Source: CAD feature listing. Evaluate the final solid. Frame: model axes, mm. Face numbers are marked on the shaded views. A direction names the side the tool comes from. Coordinates: 2 decimals unless noted, no trailing zeros. Order: outer loops, then holes, each group sorted by start corner. A loop starts at its lowest first (then second) coordinate and runs counter-clockwise, first axis right, second up. Notation, with made-up numbers: (32.5, -8.5) -> (61.5, -8.5) arc R26 cw to (61.5, 24.5) -> close; hole circle Ø5 at (13, 14). An arc over 180 degrees is marked (long way). Write each question's results on one line, items separated by ' | '. Start each with the question number.
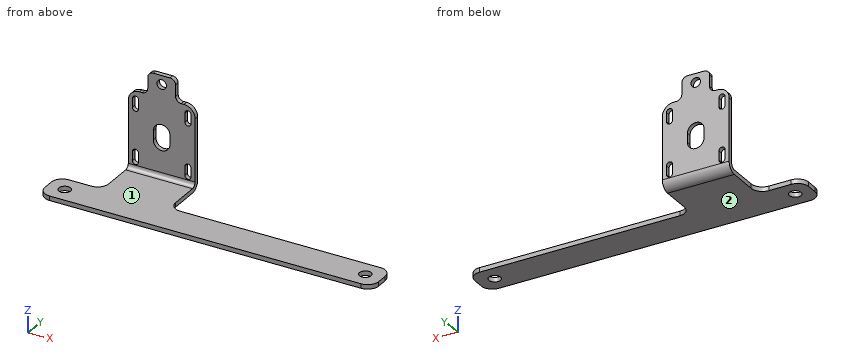
from build123d import *

# Parameters (mm, degrees)
SKETCH1_R                    = 4.25
BASE_FLANGE1_DEPTH           = 4
EDGE_FLANGE1_STRIP_W         = 24
EDGE_FLANGE1_STRIP_H         = 4
EDGE_FLANGE1_STRIP_CUT_DEPTH = 60
EDGE_FLANGE1_DEPTH           = 60
SKETCH11_R                   = 5.25
TAB1_DEPTH                   = 4
FILLET2_R                    = 10


# Sheet-metal steps are written as plain solids
with BuildPart() as part:
    # Sketch1 → Base-Flange1 (new body)
    with BuildSketch(Plane(origin=(0, 0, 0), x_dir=(1, 0, 0), z_dir=(0, 1, 0))):
        with BuildLine():
            Line((30, -35), (17.5, -35))
            ThreePointArc((17.5, -35), (13.964466094, -36.464466094), (12.5, -40))
            Line((12.5, -40), (12.5, -50))
            ThreePointArc((12.5, -50), (11.035533906, -53.535533906), (7.5, -55))
            Line((7.5, -55), (-7.5, -55))
            ThreePointArc((-7.5, -55), (-11.035533906, -53.535533906), (-12.5, -50))
            Line((-12.5, -50), (-12.5, -40))
            ThreePointArc((-12.5, -40), (-13.964466094, -36.464466094), (-17.5, -35))
            Line((-17.5, -35), (-30, -35))
            Line((-30, -35), (-30, 35))
            Line((-30, 35), (30, 35))
            Line((30, 35), (30, -35))
        make_face()
        with Locations(Location((0, -47, 0), (0, 0, 270))):
            Circle(SKETCH1_R, mode=Mode.SUBTRACT)
        with BuildLine():
            Line((-26.32, 19.57), (-26.32, 27.57))
            ThreePointArc((-26.32, 27.57), (-23.57, 30.32), (-20.82, 27.57))
            Line((-20.82, 27.57), (-20.82, 19.57))
            ThreePointArc((-20.82, 19.57), (-23.57, 16.82), (-26.32, 19.57))
        make_face(mode=Mode.SUBTRACT)
        with BuildLine():
            Line((26.32, 19.57), (26.32, 27.57))
            ThreePointArc((26.32, 27.57), (23.57, 30.32), (20.82, 27.57))
            Line((20.82, 27.57), (20.82, 19.57))
            ThreePointArc((20.82, 19.57), (23.57, 16.82), (26.32, 19.57))
        make_face(mode=Mode.SUBTRACT)
        with BuildLine():
            Line((26.32, -27.57), (26.32, -19.57))
            ThreePointArc((26.32, -19.57), (23.57, -16.82), (20.82, -19.57))
            Line((20.82, -19.57), (20.82, -27.57))
            ThreePointArc((20.82, -27.57), (23.57, -30.32), (26.32, -27.57))
        make_face(mode=Mode.SUBTRACT)
        with BuildLine():
            Line((-20.82, -27.57), (-20.82, -19.57))
            ThreePointArc((-20.82, -19.57), (-23.57, -16.82), (-26.32, -19.57))
            Line((-26.32, -19.57), (-26.32, -27.57))
            ThreePointArc((-26.32, -27.57), (-23.57, -30.32), (-20.82, -27.57))
        make_face(mode=Mode.SUBTRACT)
        with BuildLine():
            Line((7.5, 4), (7.5, -4))
            ThreePointArc((7.5, -4), (0, -11.5), (-7.5, -4))
            Line((-7.5, -4), (-7.5, 4))
            ThreePointArc((-7.5, 4), (0, 11.5), (7.5, 4))
        make_face(mode=Mode.SUBTRACT)
    extrude(amount=-BASE_FLANGE1_DEPTH)

    # Edge-Flange1 strip (across the edge) → Edge-Flange1 strip cut (cut)
    with BuildSketch(Plane(origin=(-30, -4, -35), x_dir=(0, 0, 1), z_dir=(1, 0, 0))):
        with Locations((-8, -2)):
            Rectangle(EDGE_FLANGE1_STRIP_W, EDGE_FLANGE1_STRIP_H)
    extrude(amount=EDGE_FLANGE1_STRIP_CUT_DEPTH, mode=Mode.SUBTRACT)

    # Edge-Flange1 section (across the edge) → Edge-Flange1 (add)
    with BuildSketch(Plane(origin=(-30, -4, -35), x_dir=(0, 0, 1), z_dir=(1, 0, 0))):
        with BuildLine():
            Line((-4, 4), (-4, 40))
            Line((-4, 40), (0, 40))
            Line((0, 40), (0, 4))
            ThreePointArc((0, 4), (1.171572875, 1.171572875), (4, 0))
            Line((4, 0), (4, -4))
            ThreePointArc((4, -4), (-1.656854249, -1.656854249), (-4, 4))
        make_face()
    extrude(amount=EDGE_FLANGE1_DEPTH)

    # Sketch11 → Tab1 (add)
    with BuildSketch(Plane(origin=(0, 0, -39), x_dir=(-1, 0, 0), z_dir=(0, 0, -1))):
        Polygon((-30, -44), (-230, -44), (-230, -74), (70, -74), (70, -44), (30, -44), (30, -8), (-30, -8), align=None)
        with Locations(Location((-215, -59, 0), (0, 0, 90))):
            Circle(SKETCH11_R, mode=Mode.SUBTRACT)
        with Locations(Location((55, -59, 0), (0, 0, 90))):
            Circle(SKETCH11_R, mode=Mode.SUBTRACT)
    extrude(amount=-TAB1_DEPTH)

    # Fillet2
    fillet2_edges = [part.edges().sort_by_distance(p)[0] for p in [
        (-30, -44, -37),
        (30, -44, -37),
        (-70, -44, -37),
        (-70, -74, -37),
        (230, -74, -37),
        (230, -44, -37),
        (30, -2, 35),
        (-30, -2, 35),
    ]]
    fillet(fillet2_edges, radius=FILLET2_R)


solid = part.part
(1) Line query: L1, parallel to X at y = -59, z = -37.9; L2, parallel to X at y = -2.6, z = 47; L3, parallel to Y at x = -28.5, z = 13.5. Output: solid intervals per line, ascending.
(2) Section A-A on x = 215. Return the cut outline in (y, z), then the cut area to 3 significant figures.
(3) Section D-D on y = -47.5. Return the cut outline in (x, z).
(4) Reachability of the marked faces 1 and 2 from +Z, -Z, +X, -X, +Y, -Y: full face, straight path, thin tool, end or side. Return the list, or none.
(5) Section C-C on y = -60. Return the cut outline in (x, z).
(6) First-contact query: P1, Ø1.2, axis at x = 156.5, z = -37.5, coming from the +Y side; P2, Ø4.5, axis at y = -2, z = -24.5, coming from the -X side; P3, Ø3, axis at y = -1.5, z = -22, coming from the +X side; P4, Ø12, axis at x = 215, y = -59, coming from the -Z side. Flat tips, straight axial feed; report the tip coordinate or a pass-through.
(7) Section B-B on x = 0. Return the cut outline in (y, z).
Results list:
1) L1: x = -70 to -60.25, -49.75 to 209.75, 220.25 to 230 | L2: x = -12.5 to -4.25, 4.25 to 12.5 | L3: y = -4 to 0
2) outline: (-74, -39) -> (-64.25, -39) -> (-64.25, -35) -> (-74, -35) -> close; (-53.75, -39) -> (-44, -39) -> (-44, -35) -> (-53.75, -35) -> close | area: 78.0 mm²
3) outline: (-67.6, -39) -> (227.6, -39) -> (227.6, -35) -> (-67.6, -35) -> close
4) face 1: +Z, +X, -X, -Y | face 2: -Z, +X, -X, +Y, -Y
5) outline: (-70, -39) -> (-60.15, -39) -> (-60.15, -35) -> (-70, -35) -> close; (-49.85, -39) -> (209.85, -39) -> (209.85, -35) -> (-49.85, -35) -> close; (220.15, -39) -> (230, -39) -> (230, -35) -> (220.15, -35) -> close
6) P1: stops at y = -44 | P2: stops at x = -30 | P3: stops at x = 30 | P4: stops at z = -39
7) outline: (-74, -39) -> (-8, -39) arc R8 ccw to (0, -31) -> (0, -11.5) -> (-4, -11.5) -> (-4, -31) arc R4 cw to (-8, -35) -> (-74, -35) -> close; (-4, 11.5) -> (0, 11.5) -> (0, 42.75) -> (-4, 42.75) -> close; (-4, 51.25) -> (0, 51.25) -> (0, 55) -> (-4, 55) -> close
